Build history of the part. All positions in model axes, mm. A direction names the side the tool comes from. Round coordinates to 2 decimals unless told otherwise and drop trailing zeros. Order: outer loops, then holes, each group sorted by start corner. A loop starts at its lowest first (then second) coordinate and runs counter-clockwise, first axis right, second up. Notation, with made-up numbers: (-24.75, 58) -> (15.25, 58) arc R21 cw to (15.25, 74) -> close; hole circle Ø3 at (73, 25.5). An arc over 180 degrees is marked (long way). Use a Markdown table: item, result. Add a question column.
Item 1: Slice it at C-C, the plane y = 2. Give the cut face in (x, z).
Item 2: Probe L1, parallel to Z at x = 11.5, y = 3.5; L2, parallel to Z at x = 11.5, y = 17.35; L3, parallel to Y at x = 0, z = 4. List the from-to ranges inside material, lowest first.
Item 3: Pin check, flat tips, straight feed: pin 1 (1 mm diameter, centred on x = 2, z = 9.5, fed in from -Y); pin 2 (4 mm diameter, centred on x = -10.5, z = 6.5, fed in from +Y). Stop position of each tip, or through.
Item 4: Slice it at A-A, the plane z = 6. State how many separate pieces and enclosed holes the cut face has, plus the area to 3 significant figures.
Item 5: 3-axis set-ups, long thin cutter, end or side, ignore diameter. For faces 1 (the face through (8.3, 18, 8.4)), 2 (the face through (4.715, 4.699, 6.084)), 3 (the face through (0, 20, 6)): which of +Z, -Z, +X, -X, +Y, -Y reach the whole face in a straight line?
Item 6: Slice it at D-D, the plane y = 6.5. Give the cut face in (x, z), plus the area to 3 significant figures.
Item 7: Two-plate mould, pull along Z, no slides. Class faces 4 (the face through (17.5, 10, 6)), 5 (the face through (-9.252, 7.888, 5.901)), 6 (the face through (0, 8, 0)): released by +Z, released by -Z, zero draft, split by the parting line, or undercut.
Item 8: Slice it at B-B, the plane x = 0. Give the cut face in (y, z).
from build123d import *

# Parameters (mm, degrees)
SKETCH1_R                      = 3.5
BOSS_EXTRUDE1_DEPTH            = 12
CBORE_FOR_M4_SHCS1_D           = 4.5
CBORE_FOR_M4_SHCS1_CBORE_D     = 8
CBORE_FOR_M4_SHCS1_CBORE_DEPTH = 4
FILLET1_R                      = 1


with BuildPart() as part:
    # Sketch1 → Boss-Extrude1 (new body)
    with BuildSketch(Plane.XY):
        Polygon((-17.5, 20), (17.5, 20), (17.5, 0), (5, 0), (5, 5), (-5, 5), (-5, 0), (-17.5, 0), align=None)
        with Locations((0, 12)):
            Circle(SKETCH1_R, mode=Mode.SUBTRACT)
    extrude(amount=BOSS_EXTRUDE1_DEPTH)

    # CBORE for M4 SHCS1 (through all)
    with Locations(Plane(origin=(0, 20, 0), x_dir=(1, 0, 0), z_dir=(0, 1, 0))):
        with Locations((-11.5, -6), (11.5, -6)):
            CounterBoreHole(CBORE_FOR_M4_SHCS1_D / 2, CBORE_FOR_M4_SHCS1_CBORE_D / 2, CBORE_FOR_M4_SHCS1_CBORE_DEPTH)

    # Fillet1
    fillet1_edges = [part.edges().sort_by_distance(p)[0] for p in [
        (5, 5, 6),
        (-5, 5, 6),
        (-17.5, 20, 6),
        (17.5, 20, 6),
    ]]
    fillet(fillet1_edges, radius=FILLET1_R)


solid = part.part
Check sheet entries:
| question | item | result |
|---|---|---|
| 1 | outline | (-17.5, 0) -> (-5, 0) -> (-5, 12) -> (-17.5, 12) -> close; (5, 0) -> (17.5, 0) -> (17.5, 12) -> (5, 12) -> close; hole circle Ø4.5 at (-11.5, 6); hole circle Ø4.5 at (11.5, 6) |
| 2 | L1 | 0 to 3.75, 8.25 to 12 |
| 2 | L2 | 0 to 2, 10 to 12 |
| 2 | L3 | 5 to 8.5, 15.5 to 20 |
| 3 | pin 1 | y = 5 |
| 3 | pin 2 | y = 16 |
| 4 | separate pieces | 3 |
| 4 | enclosed holes | 1 |
| 4 | area | 404 mm2 |
| 5 | face 1 | +Y |
| 5 | face 2 | +Z, -Z, -Y |
| 5 | face 3 | +Z, -Z, +X, -X, +Y |
| 6 | outline | (-17.5, 0) -> (17.5, 0) -> (17.5, 12) -> (-17.5, 12) -> close; hole circle Ø4.5 at (-11.5, 6); hole circle Ø4.5 at (11.5, 6) |
| 6 | area | 388 mm2 |
| 7 | face 4 | zero draft |
| 7 | face 5 | undercut |
| 7 | face 6 | released by -Z |
| 8 | outline | (5, 0) -> (8.5, 0) -> (8.5, 12) -> (5, 12) -> close; (15.5, 0) -> (20, 0) -> (20, 12) -> (15.5, 12) -> close |
